Autodesk Inventor part; units mm, degrees
ref_plane "YZ Plane" through (0, 0, 0) normal (1, 0, 0) x (0, 1, 0)
ref_plane "XZ Plane" through (0, 0, 0) normal (0, 1, 0) x (-1, 0, 0)
ref_plane "XY Plane" through (0, 0, 0) normal (0, 0, 1) x (1, 0, 0)
sketch "Sketch1" plane through (0, 0, 0) normal (1, 0, 0) x (0, 1, 0)
  line L0 (10, 150) -> (48, 150)
  line L1 (50, 148) -> (50, 2)
  line L2 (48, 0) -> (0, 0)
  line L3 (0, 2) -> (46, 2)
  line L4 (48, 4) -> (48, 146)
  line L5 (46, 148) -> (10, 148)
  line L6 (0, 0) -> (0, 2)
  line L7 (10, 150) -> (10, 148)
  arc A0 (48, 146) -> (46, 148) centre (46, 146) ccw
  arc A1 (50, 148) -> (48, 150) centre (48, 148) ccw
  arc A2 (48, 0) -> (50, 2) centre (48, 2) ccw
  arc A3 (46, 2) -> (48, 4) centre (46, 4) ccw
  point P0 (50, 150)
  point P1 (50, 0)
  dimension "d0" = 40
  dimension "d1" = 150
  dimension "d2" = 50
  dimension "d3" = 2
  dimension "d4" = 2
extrude "Extrusion1" add sketch "Sketch1" along normal blind 380
sketch "Sketch2" plane through (0, 50, 148) normal (0, 1, 0) x (1, 0, 0)
  line L0 (330, 108) -> (50, 108) construction
  line L1 (330, 83) -> (50, 83)
  line L2 (50, 133) -> (330, 133)
  arc A0 (330, 83) -> (330, 133) centre (330, 108) ccw
  arc A1 (50, 133) -> (50, 83) centre (50, 108) ccw
  line L3 (0, 146) -> (380, 146)
  line L4 (0, 144) -> (0, 2)
  line L5 (380, 146) -> (380, 0)
  line L6 (0, 148) -> (380, 148)
  point P0 (190, 108)
  dimension "d7" = 280
  dimension "d8" = 190
  dimension "d9" = 50
  dimension "d10" = 40
extrude "Extrusion2" cut sketch "Sketch2" against normal up to surface (2 mm away)
sketch "Sketch3" plane through (0, 0, 0) normal (0, 0, -1) x (-1, 0, 0)
  line L0 (0, 0) -> (-380, 0)
  line L1 (-380, 0) -> (-380, 48)
  point P0 (-355, 24)
  point P1 (-285, 24)
  point P2 (-190, 24)
  point P3 (-25, 24)
  point P4 (-95, 24)
  dimension "d13" = 24
  dimension "d14" = 70
  dimension "d15" = 95
  dimension "d16" = 95
  dimension "d17" = 70
  dimension "d18" = 25
hole "Hole1" at (355, 24, 0) at (285, 24, 0) at (190, 24, 0) at (25, 24, 0) at (95, 24, 0) direction (0, 0, 1) diameter 6 end through all
properties part number "SidePanelCoverSpacer"
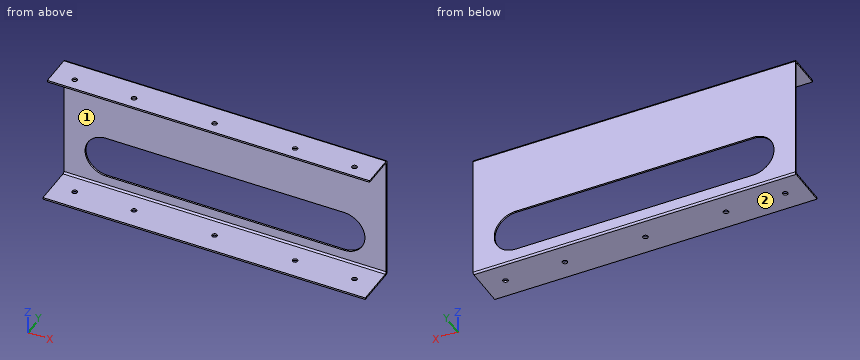
For this review, take the finished solid that the model builds, in its own axes (mm). Face numbers are marked on the shaded views. A direction names the side the tool comes from. Coordinates: 2 decimals unless noted, no trailing zeros. Order: outer loops, then holes, each group sorted by start corner. A loop starts at its lowest first (then second) coordinate and runs counter-clockwise, first axis right, second up. Notation, with made-up numbers: (15, -30) - (24, -30) arc R15 ccw to (24, -18) - close; hole circle Ø5 at (-26.5, 52.5). An arc over 180 degrees is marked (long way). Use one line per item in the form item = value.
Q1. Consider section D-D (y = 6). Give the boundary of the cut face in (x, z).
Checked values:
outline = (0, 0) - (380, 0) - (380, 2) - (0, 2) - close
Q2. Consider section C-C (z = 40). Give the boundary of the cut face in (x, y), then the cut area to 3 significant figures.
Checked values:
outline = (0, 48) - (25, 48) - (25, 50) - (0, 50) - close; (355, 48) - (380, 48) - (380, 50) - (355, 50) - close
area = 100 mm2
Q3. Consider section B-B (x = 62.5). Give the boundary of the cut face in (y, z), then the cut area to 3 significant figures.
Checked values:
outline = (0, 0) - (48, 0) arc R2 ccw to (50, 2) - (50, 15) - (48, 15) - (48, 4) arc R2 cw to (46, 2) - (0, 2) - close; (10, 148) - (46, 148) arc R2 cw to (48, 146) - (48, 65) - (50, 65) - (50, 148) arc R2 ccw to (48, 150) - (10, 150) - close
area = 372 mm2
Q4. For probe 1 along X at (y, z) = (24, 1.45); probe 2 along Z at (x, y) = (218, 46.5); probe 3 along Z at (x, y) = (281, 19.5), list the stretches that pass through material, from the lowest coordinate up. Write a range as from..to.
Checked values:
probe_1 = 0..22, 28..92, 98..187, 193..282, 288..352, 358..380
probe_2 = 0..2.06, 147.94..150
probe_3 = 0..2, 148..150
Q5. For the marked faces 1 and 2, list the 3-axis set-ups (+Z, -Z, +X, -X, +Y, -Y) from which the entire face can be reached by the end or side of a thin tool; tool diameter is ignored.
Checked values:
face_1 = +X, -X, -Y
face_2 = -Z, +X, -X, +Y, -Y
Q6. For P1, Ø0.6, axis at x = 165.5, y = 48.5, coming from the -Z side; P2, Ø1, axis at x = 147.5, y = 49, coming from the +Z side; P3, Ø12, axis at x = 127.5, z = 87.5, coming from the -Y side, all flat-tipped, find the tip position at first contact; note any pin that passes through.
Checked values:
P1 = 0.01
P2 = 149.94
P3 = 48
Q7. Consider section A-A (y = 40). Give the boundary of the cut face in (x, z).
Checked values:
outline = (0, 0) - (380, 0) - (380, 2) - (0, 2) - close; (0, 148) - (380, 148) - (380, 150) - (0, 150) - close
